Input: part model. Units: mm. Frame: model coordinates. A direction names the side the tool comes from. Round coordinates to 2 decimals unless told otherwise and drop trailing zeros. Order: outer loops, then holes, each group sorted by start corner. A loop starts at its lowest first (then second) coordinate and runs counter-clockwise, first axis right, second up. Notation, with made-up numbers: (52, -34.75) -> (90, -34.75) arc R24 ccw to (90, 3.25) -> close; hole circle Ø11 at (-22.75, 50.5). An arc over 180 degrees is marked (long way). Answer as CSV lines item,"result". Start each with the question number.
1) Line query: L1, parallel to X at y = -11.25, z = -34.5; L2, parallel to Z at x = -19.5, y = -15.5; L3, parallel to X at y = -10, z = 15.5. Output: solid intervals per line, ascending.
2) Section query D-D, the plane x = -47. Output: boundary loops of the cut face in (y, z), and give its area (3 significant figures).
3) First-contact query: P1, Ø3, axis at y = -7.5, z = 28.5, coming from the -X side; P2, Ø3, axis at x = -35.5, y = -8, coming from the -Z side; P3, Ø12, axis at x = -17, y = -4.5, coming from the +Z side; P4, Ø17, axis at x = -27.64, z = 28.92, coming from the -Y side. Flat tips, straight axial feed; report the tip coordinate or a pass-through.
4) Section query A-A, the plane x = -16. Output: boundary loops of the cut face in (y, z), and give its area (3 significant figures).
5) Section query B-B, the plane y = -10. Output: boundary loops of the cut face in (x, z), and give its area (3 significant figures).
6) Access query for faces 4 (the face through (0, -15, -40)), 5 (the face through (1.33, -14.79, -44.79)). Directions: +Z, -Z, +X, -X, +Y, -Y. A direction counts if a zero-diameter tool reaches every point of the face in a straight line with its end or side. Return the directions, or none.
7) Mould query, pull axis X, two halves, no side actions, for faces 1 (the face through (0, -15, 40)), 2 (the face through (-56.99, -14.79, 1.09)), 3 (the face through (56.994, -14.79, 0.819)). Classes: +X half, -X half, draft (parallel to the pull), parting line (faces both ways), or undercut.
8) Section query C-C, the plane z = 49. Output: boundary loops of the cut face in (x, y).
```python
from build123d import *

# Parameters (mm, degrees)
F1_DEPTH = 30


with BuildPart() as f1:
    # F0 (on Front) → F1 (new body)
    with BuildSketch(Plane.XZ):
        with BuildLine():
            ThreePointArc((11.976271, 55.727632), (0.118423, 47.051717), (-11.695602, 55.787211))
            ThreePointArc((-11.695602, 55.787211), (-57, 0), (-11.695602, -55.787211))
            ThreePointArc((-11.695602, -55.787211), (1.58817, -44.777874), (15.618535, -54.81844))
            ThreePointArc((15.618535, -54.81844), (56.969087, 1.877013), (11.976271, 55.727632))
        make_face()
        with BuildLine():
            ThreePointArc((32.547889, 23.251558), (38.09144, 12.208285), (40, 0))
            ThreePointArc((40, 0), (38.09144, -12.208285), (32.547889, -23.251558))
            ThreePointArc((32.547889, -23.251558), (34.457846, -25.803765), (35.135292, -28.91869))
            ThreePointArc((35.135292, -28.91869), (30.096884, -36.00322), (21.751142, -33.56915))
            ThreePointArc((21.751142, -33.56915), (0, -40), (-21.751142, -33.56915))
            ThreePointArc((-21.751142, -33.56915), (-32.816909, -34.340945), (-32.547889, -23.251558))
            ThreePointArc((-32.547889, -23.251558), (-40, 0), (-32.547889, 23.251558))
            ThreePointArc((-32.547889, 23.251558), (-32.816909, 34.340945), (-21.751142, 33.56915))
            ThreePointArc((-21.751142, 33.56915), (0, 40), (21.751142, 33.56915))
            ThreePointArc((21.751142, 33.56915), (30.096884, 36.00322), (35.135292, 28.91869))
            ThreePointArc((35.135292, 28.91869), (34.457846, 25.803765), (32.547889, 23.251558))
        make_face(mode=Mode.SUBTRACT)
    extrude(amount=F1_DEPTH)


solid = f1.part
```
Findings:
1,L1,"x = -45.37 to -32.65, -22.63 to -20.24, 20.24 to 22.63, 32.65 to 45.37"
1,L2,"z = -53.56 to -34.92, 34.92 to 53.56"
1,L3,"x = -54.85 to -36.87, 36.87 to 54.85"
2,outline,"(-30, -32.25) -> (0, -32.25) -> (0, 32.25) -> (-30, 32.25) -> close"
2,area,"1,930 mm^2"
3,P1,"stops at x = -50.2"
3,P2,"stops at z = -45.75"
3,P3,"stops at z = 55.79"
3,P4,"stops at y = -30"
4,outline,"(-30, -54.71) -> (0, -54.71) -> (0, -36.66) -> (-30, -36.66) -> close; (-30, 36.66) -> (0, 36.66) -> (0, 54.71) -> (-30, 54.71) -> close"
4,area,"1,080 mm^2"
5,outline,"(-11.7, -55.79) arc R14.13 cw to (15.62, -54.82) arc R57 ccw to (11.98, 55.73) arc R12.4 cw to (-11.7, 55.79) arc R57 ccw to start; hole (-32.55, -23.25) arc R7.5 ccw (long way) to (-21.75, -33.57) arc R40 ccw to (21.75, -33.57) arc R7.5 ccw to (35.14, -28.92) arc R7.5 ccw to (32.55, -23.25) arc R40 ccw to (40, 0) arc R40 ccw to (32.55, 23.25) arc R7.5 ccw to (35.14, 28.92) arc R7.5 ccw to (21.75, 33.57) arc R40 ccw to (-21.75, 33.57) arc R7.5 ccw (long way) to (-32.55, 23.25) arc R40 ccw to start"
5,area,"4,400 mm^2"
6,face 4,"+Y, -Y"
6,face 5,"-Z, +Y, -Y"
7,face 1,"undercut"
7,face 2,"-X half"
7,face 3,"+X half"
8,outline,"(-29.12, -30) -> (-6.52, -30) -> (-6.52, 0) -> (-29.12, 0) -> close; (6.82, -30) -> (29.12, -30) -> (29.12, 0) -> (6.82, 0) -> close"
